Autodesk Inventor part; units mm, degrees
ref_plane "YZ Plane" through (0, 0, 0) normal (1, 0, 0) x (0, 1, 0)
ref_plane "XZ Plane" through (0, 0, 0) normal (0, 1, 0) x (-1, 0, 0)
ref_plane "XY Plane" through (0, 0, 0) normal (0, 0, 1) x (1, 0, 0)
sketch "スケッチ1" plane through (0, 0, 0) normal (0, 0, 1) x (1, 0, 0)
  circle A0 centre (-21.6908, -16.4118) radius 19.1 construction
  circle A1 centre (-58.0056, -24.4791) radius 22.1 construction
  circle A2 centre (-105.5257, -16.4118) radius 30.1 construction
  circle A3 centre (-122.6945, 30.2622) radius 1.5
  circle A4 centre (-75.5257, 23.124) radius 1.5
  circle A5 centre (-65.5257, -10.4118) radius 1.5
  circle A6 centre (-145.5257, 0.5882) radius 1.5
  circle A7 centre (-105.5257, -16.4118) radius 7.025
  circle A8 centre (-21.6908, -16.4118) radius 1.5
  arc A9 (-17.8785, -18.8026) -> (-19.2493, -12.6317) centre (-21.6908, -16.4118) ccw
  arc A10 (-61.0009, -47.384) -> (-50.9717, -46.4821) centre (-58.0056, -24.4791) ccw
  circle A11 centre (-34.2292, -36.4056) radius 1.5
  circle A12 centre (-41.5152, -3.6073) radius 1.5
  arc A13 (-39.0737, 0.1727) -> (-41.3386, 0.8892) centre (-41.5152, -3.6073) ccw
  arc A14 (-32.8589, -40.6919) -> (-30.4168, -38.7963) centre (-34.2292, -36.4056) ccw
  circle A15 centre (-79.2726, -40.4563) radius 1.5
  circle A16 centre (-79.2726, -40.4563) radius 4.5
  line L0 (-17.8785, -18.8026) -> (-30.4168, -38.7963)
  line L1 (-32.8589, -40.6919) -> (-50.9717, -46.4821)
  line L2 (-19.2493, -12.6317) -> (-39.0737, 0.1727)
  arc A17 (-149.0922, 3.3323) -> (-149.4523, -1.6098) centre (-145.5257, 0.5882) ccw
  line L3 (-149.4523, -1.6098) -> (-132.6633, -31.6026)
  line L4 (-102.3494, -47.3492) -> (-78.813, -44.9328)
  line L5 (-61.0009, -47.384) -> (-79.8561, -44.9183)
  circle A18 centre (-72.8083, -2.3784) radius 1.5
  arc A19 (-72.6317, 2.1181) -> (-76.944, -4.1523) centre (-72.8083, -2.3784) ccw
  line L6 (-41.3386, 0.8892) -> (-72.6317, 2.1181)
  arc A20 (-61.4337, -12.2841) -> (-61.2133, -9.1259) centre (-65.5257, -10.4118) ccw
  line L7 (-61.4337, -12.2841) -> (-75.1806, -42.3286)
  arc A21 (-82.5911, -37.417) -> (-76.944, -4.1523) centre (-105.5257, -16.4118) ccw
  arc A22 (-132.6633, -31.6026) -> (-102.3494, -47.3492) centre (-105.5257, -16.4118) ccw
  arc A23 (-122.0212, 34.7115) -> (-126.261, 33.0062) centre (-122.6945, 30.2622) ccw
  arc A24 (-71.2133, 24.4099) -> (-74.8523, 27.5733) centre (-75.5257, 23.124) ccw
  line L8 (-126.261, 33.0062) -> (-149.0922, 3.3323)
  line L9 (-122.0212, 34.7115) -> (-74.8523, 27.5733)
  line L10 (-71.2133, 24.4099) -> (-61.2133, -9.1259)
  circle A25 centre (-58.0056, -24.4791) radius 1.5
  point P0 (0, 0)
  point P1 (0, 0)
  dimension "d0" = 14.05
  dimension "d1" = 3
  dimension "d2" = 3
  dimension "d3" = 1
  dimension "d4" = 3
  dimension "d5" = 3
  dimension "d6" = 3
  dimension "d7" = 3
  dimension "d8" = 3
  dimension "d9" = 3
  dimension "d10" = 9
  dimension "d11" = 3
  dimension "d12" = 3
  dimension "d13" = 9
  dimension "d14" = 31.1
  dimension "d15" = 31.1
  dimension "d16" = 9
  dimension "d17" = 9
  dimension "d18" = 3
extrude "押し出し1" add sketch "スケッチ1" along normal blind 3 contours L0 A14 L1 A10 L5 L4 A16 L7 A20 L10 L6 A13 L2 A9 | L10 A20 L7 A16 A21 A19 L6 | L5 A16 L4 | A16
sketch "スケッチ2" plane through (0, 0, 0) normal (0, 0, -1) x (-1, 0, 0)
  circle A0 centre (58.0056, -24.4791) radius 1.5
  circle A1 centre (72.8083, -2.3784) radius 1.5
  circle A2 centre (41.5152, -3.6073) radius 1.5
  circle A3 centre (34.2292, -36.4056) radius 1.5
  circle A4 centre (21.6908, -16.4118) radius 1.5
  circle A5 centre (65.5257, -10.4118) radius 1.5
  circle A6 centre (79.2726, -40.4563) radius 1.5
  arc A7 (79.8561, -44.9183) -> (82.5911, -37.417) centre (79.2726, -40.4563) ccw
  arc A8 (76.944, -4.1523) -> (82.5911, -37.417) centre (105.5257, -16.4118) ccw
  arc A9 (76.944, -4.1523) -> (72.6317, 2.1181) centre (72.8083, -2.3784) ccw
  line L0 (41.3386, 0.8892) -> (72.6317, 2.1181)
  arc A10 (41.3386, 0.8892) -> (39.0737, 0.1727) centre (41.5152, -3.6073) ccw
  line L1 (19.2493, -12.6317) -> (39.0737, 0.1727)
  arc A11 (19.2493, -12.6317) -> (17.8785, -18.8026) centre (21.6908, -16.4118) ccw
  line L2 (30.4168, -38.7963) -> (17.8785, -18.8026)
  arc A12 (30.4168, -38.7963) -> (32.8589, -40.6919) centre (34.2292, -36.4056) ccw
  line L3 (50.9717, -46.4821) -> (32.8589, -40.6919)
  arc A13 (50.9717, -46.4821) -> (61.0009, -47.384) centre (58.0056, -24.4791) ccw
  line L4 (79.8561, -44.9183) -> (61.0009, -47.384)
  circle A14 centre (65.5257, -10.4118) radius 3.5
  point P0 (0, 0)
  dimension "d21" = 7
extrude "押し出し2" cut sketch "スケッチ2" against normal blind 10 contours A14
properties part number "後ろ脚内フレーム" material "アルミニウム 7075"
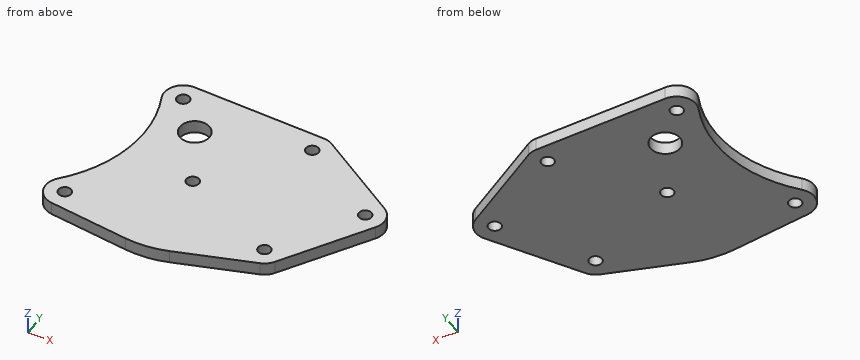
Input: part model. Units: mm. Frame: model coordinates. Coordinates: 2 decimals unless noted, no trailing zeros. Order: outer loops, then holes, each group sorted by start corner. A loop starts at its lowest first (then second) coordinate and runs counter-clockwise, first axis right, second up. Notation, with made-up numbers: M 17,83.5 L 30,83.5 A19 cw 30,93.5 Z; hole C -34,61.25 d1. An arc over 180 degrees is marked long. Write item = value, one per line. Start each with the question number.
(1) Line query: line 1 along X through (y, z) = (-3, 2.5); line 2 along Y through (x, z) = (-33, 1.5); line 3 along Y through (x, z) = (-64, 2.35). Output: solid intervals per line, ascending. Write a range as [from, to].
(2) Section D-D on y = -27. Output: boundary loops of the cut face in (x, z), and give its area (3 significant figures).
(3) Section B-B on z = 1.3. Output: boundary loops of the cut face in (x, y).
(4) First-contact query: P1, Ø4, axis at x = -29, y = -33.5, coming from the -Z side; P2, Ø1.5, axis at x = -51, z = 1, coming from the -Y side. Flat tips, straight axial feed; report the tip coordinate or a pass-through.
(5) Section C-C on x = -58.5. Output: boundary loops of the cut face in (y, z).
(6) Section A-A on x = -21.5. Output: boundary loops of the cut face in (y, z).
Result set:
q1.line_1 = [-77.27, -74.17], [-71.44, -42.89], [-40.14, -34.16]
q1.line_2 = [-40.74, -37.27], [-35.55, -3.75]
q1.line_3 = [-46.99, -13.56], [-7.26, 1.78]
q2.outline = M -76.28,0 L -23.02,0 L -23.02,3 L -76.28,3 Z
q2.area = 160 mm²
q3.outline = M -82.59,-37.42 A4.5 ccw -79.86,-44.92 L -61,-47.38 A23.1 ccw -50.97,-46.48 L -32.86,-40.69 A4.5 ccw -30.42,-38.8 L -17.88,-18.8 A4.5 ccw -19.25,-12.63 L -39.07,0.17 A4.5 ccw -41.34,0.89 L -72.63,2.12 A4.5 ccw -76.94,-4.15 A31.1 cw Z; hole C -79.27,-40.46 d3; hole C -72.81,-2.38 d3; hole C -65.53,-10.41 d7; hole C -58.01,-24.48 d3; hole C -41.52,-3.61 d3; hole C -34.23,-36.41 d3; hole C -21.69,-16.41 d3
q4.P1 = 0
q4.P2 = -46.72
q5.outline = M -47.57,0 L -25.9,0 L -25.9,3 L -47.57,3 Z; M -23.06,0 L 1.56,0 L 1.56,3 L -23.06,3 Z
q6.outline = M -24.58,0 L -17.9,0 L -17.9,3 L -24.58,3 Z; M -14.92,0 L -11.18,0 L -11.18,3 L -14.92,3 Z
